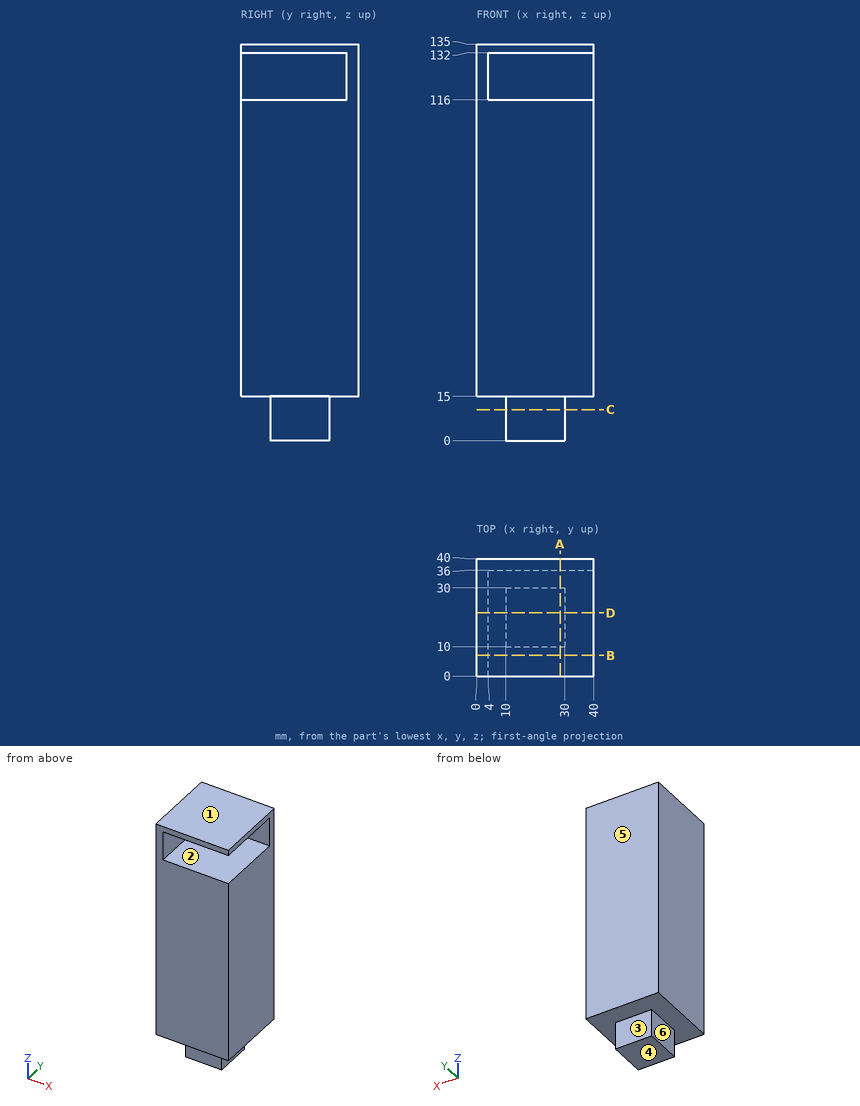
The figure shows three views and two pictorial views of one solid part (mm, origin at its lowest corner). Answer the questions. A direction names the side the tool comes from. Coordinates: 2 decimals unless noted, no trailing zeros. Loops run counter-clockwise (first coordinate to the right, second up) from the corner with the lowest first, then second, coordinate; pieces in that order, holes last.
1) Find section B-B on y = 7. Write down the section's boundary in (x, z), then the cut area to 3 significant figures.
2) Find section D-D on y = 21.5. Write down the section's boundary in (x, z), then the cut area to 3 significant figures.
3) A tool of negligible diameter and unlimited length cuts with its end or side. For the marked faces 5 and 6, from which of +Z, -Z, +X, -X, +Y, -Y can it reach the whole face along a straight path? Write none if from no direction.
4) Determine the mould class of the marked faces 1, 2, 3 and 4 for opening direction Z: pulls with the +Z half, pulls with the -Z half, needs draft (parallel to the pull), parting line crosses it, or undercut.
5) Find section C-C on z = 10.5. Write down the section's boundary in (x, y).
6) Find the intervals of material crossed by L1, parallel to Z at x = 18, y = 33.5; L2, parallel to Z at x = 15.5, y = 24.5; L3, parallel to Y at x = 13, z = 122, in increasing order.
7) Find section A-A on x = 28.5. Write down the section's boundary in (y, z), then the cut area to 3 significant figures.
8) Flat-ended cylindrical pins translate along their axes: pin 1 Ø4.5 at (y, z) = (22, 6.5) entering from -X; pin 2 Ø4.5 at (x, z) = (16.5, 4.5) entering from +Y; pin 3 Ø5 at (y, z) = (18, 128) entering from +X. Find the tip coordinate at first contact, or state that the pin passes through.
Values:
1. outline: (0, 15) - (40, 15) - (40, 116) - (4, 116) - (4, 132) - (40, 132) - (40, 135) - (0, 135) - close
1. area: 4,220 mm2
2. outline: (0, 15) - (10, 15) - (10, 0) - (30, 0) - (30, 15) - (40, 15) - (40, 116) - (4, 116) - (4, 132) - (40, 132) - (40, 135) - (0, 135) - close
2. area: 4,520 mm2
3. face 5: +Z, -Z, +X, -X, +Y
3. face 6: -Z, -X, +Y, -Y
4. face 1: pulls with the +Z half
4. face 2: undercut
4. face 3: needs draft
4. face 4: pulls with the -Z half
5. outline: (10, 10) - (30, 10) - (30, 30) - (10, 30) - close
6. L1: z = 15 to 116, 132 to 135
6. L2: z = 0 to 116, 132 to 135
6. L3: y = 36 to 40
7. outline: (0, 15) - (10, 15) - (10, 0) - (30, 0) - (30, 15) - (40, 15) - (40, 135) - (0, 135) - (0, 132) - (36, 132) - (36, 116) - (0, 116) - close
7. area: 4,520 mm2
8. pin 1: stops at x = 10
8. pin 2: stops at y = 30
8. pin 3: stops at x = 4
